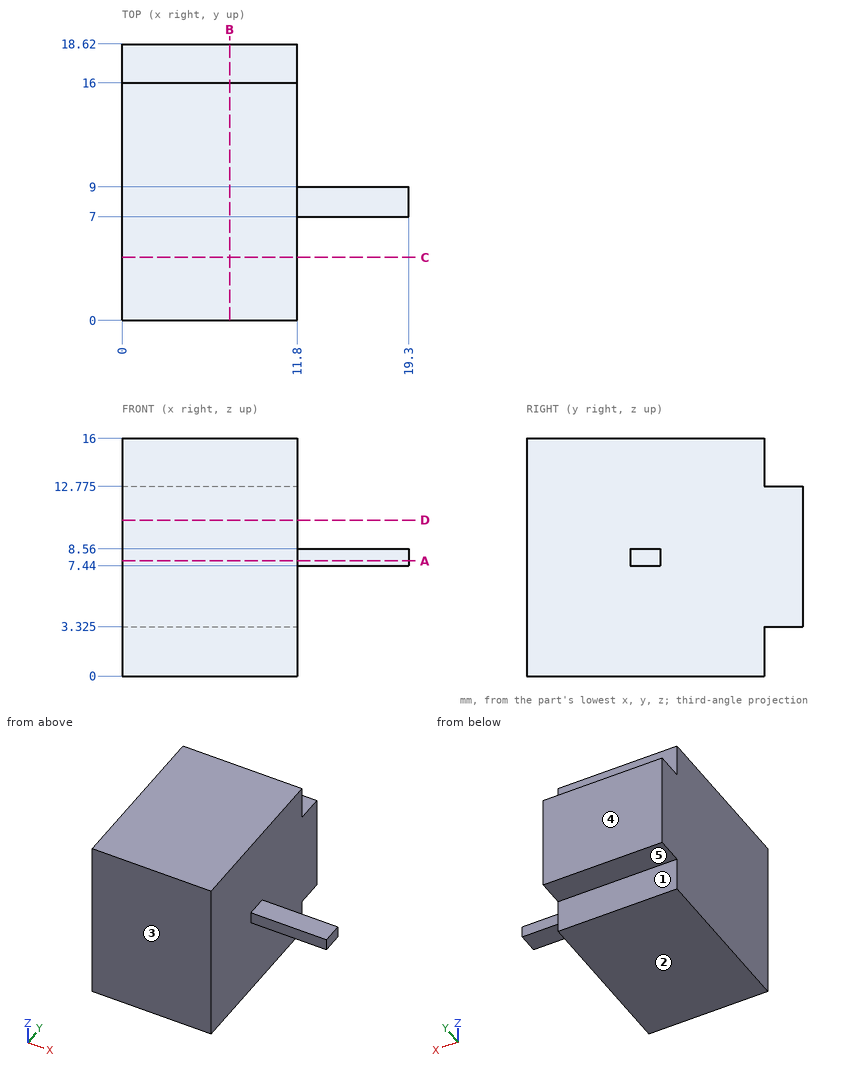
Source: three-view drawing plus pictorial views. Frame: mm from the lowest corner of the part. A direction names the side the tool comes from. Round coordinates to 2 decimals unless told otherwise and drop trailing zeros. Loops run counter-clockwise (first coordinate to the right, second up) from the corner with the lowest first, then second, coordinate; pieces in that order, holes last.
1. Mould query, pull axis Y, two halves, no side actions, for the marked faces 1, 2 and 3. Classes: released by +Y, released by -Y, zero draft, split by the parting line, or undercut.
2. Section query A-A on z = 7.75. Output: boundary loops of the cut face in (x, y), and give its area (3 significant figures).
3. Section query B-B on x = 7.25. Output: boundary loops of the cut face in (y, z) (3 decimals).
4. Contact query for flat-ended pins moving along their axis: pin 1 (1 mm diameter, centred on x = 4, z = 1.5, fed in from +Y); pin 2 (2 mm diameter, centred on x = 14.5, y = 7.5, fed in from -Z); pin 3 (1.6 mm diameter, centred on x = 15, y = 8, fed in from +Z). Output: stop coordinate, or through.
5. Section query C-C on y = 4.25. Output: boundary loops of the cut face in (x, z), and give its area (3 significant figures).
6. Access query for the marked faces 4 and 5. Directions: +Z, -Z, +X, -X, +Y, -Y. A direction counts if a zero-diameter tool reaches every point of the face in a straight line with its end or side. Return the directions, or none.
7. Ray query, L1, parallel to X at y = 6.25, z = 14.75; L2, parallel to Y at x = 1.5, z = 1; L3, parallel to Z at x = 13.5, y = 7.5. Return the intervals inside material, ascending.
8. Section query D-D on z = 10.5. Output: boundary loops of the cut face in (x, y), and give its area (3 significant figures).
Answers below:
1. face 1: released by +Y
1. face 2: zero draft
1. face 3: released by -Y
2. outline: (0, 0) - (11.8, 0) - (11.8, 7) - (19.3, 7) - (19.3, 9) - (11.8, 9) - (11.8, 18.62) - (0, 18.62) - close
2. area: 235 mm2
3. outline: (0, 0) - (16, 0) - (16, 3.325) - (18.62, 3.325) - (18.62, 12.775) - (16, 12.775) - (16, 16) - (0, 16) - close
4. pin 1: stops at y = 16
4. pin 2: stops at z = 7.44
4. pin 3: stops at z = 8.56
5. outline: (0, 0) - (11.8, 0) - (11.8, 16) - (0, 16) - close
5. area: 189 mm2
6. face 4: +Z, -Z, +X, -X, +Y
6. face 5: -Z, +X, -X, +Y
7. L1: x = 0 to 11.8
7. L2: y = 0 to 16
7. L3: z = 7.44 to 8.56
8. outline: (0, 0) - (11.8, 0) - (11.8, 18.62) - (0, 18.62) - close
8. area: 220 mm2
